Here's the drawing with two shaded views (mm, measured from the low corner). I have some questions. A direction names the side the tool comes from. Give positions to 0.01 mm unless a question says otherwise; leave off trailing zeros. Loops run counter-clockwise (first coordinate to the right, second up) from the corner with the lowest first, then second, coordinate; pieces in that order, holes last.
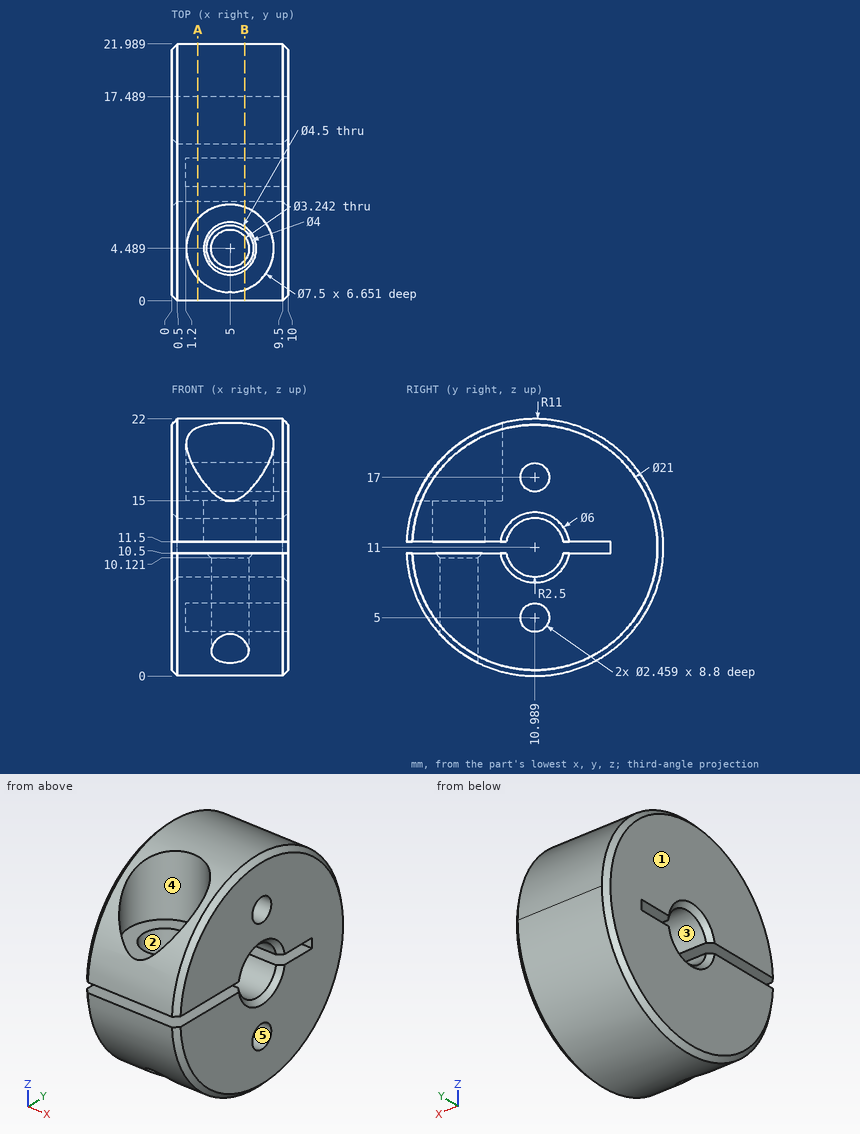
(1) Suppose I cut it at B-B on x = 6.25. Give the number of separate pieces and of enclosed holes in the cut face, plus the area to 3 significant figures.
Returned:
separate pieces: 3
enclosed holes: 2
area: 276 mm2
(2) Thinking about a two-plate mould opening in Y: for the marked faces 1 and 2, which applies, pulls with the +Y half, pulls with the -Y half, needs draft (parallel to the pull), parting line crosses it, or undercut?
Returned:
face 1: needs draft
face 2: undercut
(3) Will these pins go through, and if not, where does the flat tip stop? P1, Ø2, axis at y = 10.99, z = 17, coming from the +X side; P2, Ø2, axis at y = 10.5, z = 17, coming from the +X side; P3, Ø1.5, axis at x = 7.5, y = 9.5, coming from the +Z side (1 decimal); P4, Ø2, axis at x = 5, y = 15.5, coming from the -Z side (1 decimal).
Returned:
P1: stops at x = 1.2
P2: stops at x = 10
P3: stops at z = 22
P4: stops at z = 0.6
(4) Suppose I cut it at A-A on x = 2.25. List the corners of the cut face in (y, z) for me, plus the area to 3 significant figures.
Returned:
outline: (0, 10.5) arc R11 ccw (long way) to (7.04, 21.27) - (7.04, 15) - (1.94, 15) - (1.94, 17.25) arc R11 ccw to (0, 11.5) - (8.54, 11.5) arc R2.5 cw to (13.44, 11.5) - (17.49, 11.5) - (17.49, 10.5) - (13.44, 10.5) arc R2.5 cw to (8.54, 10.5) - close; hole circle Ø2.46 at (10.99, 5); hole circle Ø2.46 at (10.99, 17)
area: 315 mm2
(5) Which directions (+Z, -Z, +X, -X, +Y, -Y) give clear straight access to the entire face, cutting with the end or side of a thin tool? Please do the marked faces 3, 4 and 5.
Returned:
face 3: +X, -X
face 4: +Z
face 5: +X
(6) Please list where these lines run through material, in increasing order: probe 1 along Z at (x, y) = (7.25, 11); probe 2 along Z at (x, y) = (9, 11.5); probe 3 along X at (y, z) = (4, 5.5) (1 decimal).
Returned:
probe 1: z = 0 to 3.77, 6.23 to 8.5, 13.5 to 15.77, 18.23 to 22
probe 2: z = 0.01 to 3.88, 6.12 to 8.55, 13.45 to 15.88, 18.12 to 21.99
probe 3: x = 0 to 3.5, 6.5 to 10
